Answer from the drawing. Dimensions are ordinates in mm from the lowest x, y and z of the part. Round coordinates to 2 decimals unless told otherwise and drop trailing zeros. Write each loop counter-clockwise with the first axis right and the second up, starting at its lowest first coordinate (ties: lowest second). Pieces come first, ordered by that corner, then holes. Notation, with made-up numbers: (-26, 17) -> (28, 17) arc R25 ccw to (28, 41) -> close; hole circle Ø9 at (74, -9.75). An arc over 180 degrees is marked (long way). Return JSON: item names as keys, results as strings. Group by question number.
(1) Straight lines are drawn through the part: line 1 (X direction, y = 16, z = 0.9); line 2 (X direction, y = 15.25, z = 0.5); line 3 (X direction, y = 3, z = 0.4). For each, find the intervals that lie inside material, in ascending order.
(2) A cutting plane is placed at A-A on z = 0.7. Give the vertices of the cut face in (x, y) (3 decimals).
(3) A cutting plane is placed at C-C on y = 28. Give the vertices of the cut face in (x, z), then the cut area to 3 significant figures.
(4) A cutting plane is placed at B-B on y = 10.25. Give the vertices of the cut face in (x, z) (3 decimals), then the cut area to 3 significant figures.
(5) Given pin 1 (6 mm diameter, centred on x = 32.5, y = 15, fed in from -Z), flat-ended and moving along its own axis, determine where the tip first touches the part or whether it passes through.
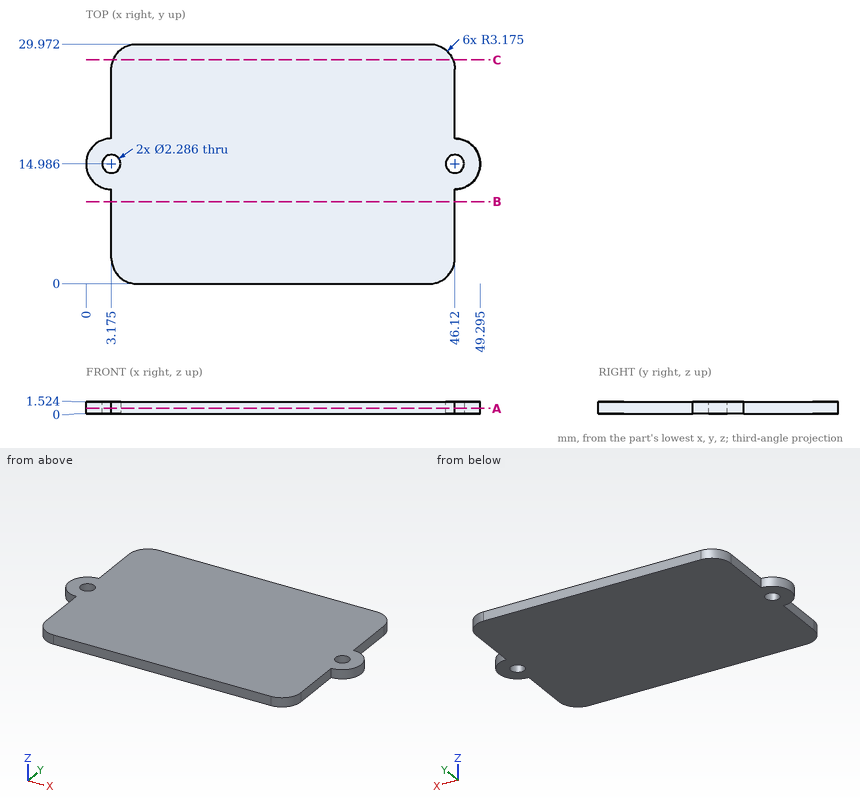
Checks:
{
 "1": {"line 1": "x = 0.17 to 2.65, 3.7 to 45.59, 46.65 to 49.13", "line 2": "x = 0.01 to 2.06, 4.29 to 45.01, 47.23 to 49.28", "line 3": "x = 3.18 to 46.12"},
 "2": {"outline": "(3.175, 3.175) arc R3.175 ccw to (6.35, 0) -> (42.945, 0) arc R3.175 ccw to (46.12, 3.175) -> (46.12, 11.811) arc R3.175 ccw to (46.12, 18.161) -> (46.12, 26.797) arc R3.175 ccw to (42.945, 29.972) -> (6.35, 29.972) arc R3.175 ccw to (3.175, 26.797) -> (3.175, 18.161) arc R3.175 ccw to (3.175, 11.811) -> close; hole circle Ø2.286 at (3.175, 14.986); hole circle Ø2.286 at (46.12, 14.986)"},
 "3": {"outline": "(3.41, 0) -> (45.88, 0) -> (45.88, 1.52) -> (3.41, 1.52) -> close", "area": "64.7 mm^2"},
 "4": {"outline": "(3.175, 0) -> (46.12, 0) -> (46.12, 1.524) -> (3.175, 1.524) -> close", "area": "65.4 mm^2"},
 "5": {"pin 1": "stops at z = 0"}
}
